Design review of the part built by this model. Coordinates are the model's own, in mm. A direction names the side the tool comes from. Round coordinates to 2 decimals unless told otherwise and drop trailing zeros. Loops run counter-clockwise (first coordinate to the right, second up) from the corner with the lowest first, then second, coordinate; pieces in that order, holes last. Notation, with made-up numbers: (-33.5, -32) - (-27.5, -32) arc R27 ccw to (-27.5, -6) - close; hole circle Ø1 at (32, 69.5). An arc over 180 degrees is marked (long way). Use one line per item in the form item = value. Start each with the question number.
(1) For pin 1 (3 mm diameter, centred on y = -1, z = -6, fed in from -X); pin 2 (2 mm diameter, centred on x = -0.5, z = -5, fed in from -Y); pin 3 (1.9 mm diameter, centred on x = 0, y = 0.5, fed in from +Z); pin 4 (1.1 mm diameter, centred on x = -0.5, z = 2, fed in from -Y), all flat-tipped, find the tip position at first contact; note any pin that passes through.
(2) Wall thickness on probe 1 along Z at (x, y) = (-3, -1); probe 2 along Z at (x, y) = (0.5, -0.75); probe 3 along Y at (x, z) = (-0.75, -18.5): over which ranges is each line inside the solid? List them lowest first. Write a range as [from, to].
(3) We need section B-B, the plane z = -22. Write out the cut boundary in (x, y).
(4) The part is to be moulded in two halves that separate along Y. For faces 1 (the cylindrical face through (-0.455, -3.463, 1.882)), 2 (the flat face through (-1.75, 1.03, 3.68)), 3 (the flat face through (0, 0, 1.27)), 4 (the flat face through (2, 2, 0)), say which applies: released by +Y, released by -Y, zero draft, split by the parting line, or undercut.
(5) Machinability: for faces 5 (the flat face through (1.64, 0.97, 2.4)), 6 (the flat face through (0, 0, -43.561)), 7 (the cylindrical face through (-0.31, 2.33, -21.48)), which of the approach directions +Z, -Z, +X, -X, +Y, -Y give a long, thin tool a straight path to every point of the face, cutting with its end or side? Answer none if there is none.
Autodesk Inventor part; units mm, degrees
ref_plane "YZ Plane" through (0, 0, 0) normal (1, 0, 0) x (0, 1, 0)
ref_plane "XZ Plane" through (0, 0, 0) normal (0, 1, 0) x (-1, 0, 0)
ref_plane "XY Plane" through (0, 0, 0) normal (0, 0, 1) x (1, 0, 0)
sketch "Sketch1" plane through (0, 0, 0) normal (0, 0, 1) x (1, 0, 0)
  circle A0 centre (0, 0) radius 3.4925
  circle A1 centre (0, 0) radius 2.3495
  line L0 (2.1997, 0) -> (1.0999, -1.905)
  line L1 (1.0999, -1.905) -> (-1.0999, -1.905)
  line L2 (-1.0999, -1.905) -> (-2.1997, 0)
  line L3 (-2.1997, 0) -> (-1.0999, 1.905)
  line L4 (-1.0999, 1.905) -> (1.0999, 1.905)
  line L5 (1.0999, 1.905) -> (2.1997, 0)
  dimension "d0" = 6.985
  dimension "d1" = 4.699
  dimension "d2" = 3.81
extrude "Extrusion1" add sketch "Sketch1" along normal blind 3.81 contours A0 | A1
extrude "Extrusion2" add sketch "Sketch1" against normal blind 43.561 contours A1 | L0 L1 L2 L3 L4 L5
extrude "Extrusion3" add sketch "Sketch1" along normal blind 1.27 contours L0 L1 L2 L3 L4 L5
thread "Thread1"
chamfer "Chamfer1" distance 0.254 angle 45 8 edges at (-3.4925, 0, 3.81) (-3.4925, 0, 0) (-1.6498, 0.9525, 3.81) (-1.6498, -0.9525, 3.81) (0, -1.905, 3.81) (1.6498, -0.9525, 3.81) (1.6498, 0.9525, 3.81) (0, 1.905, 3.81)
properties part number "Gearbox Hex Machine Screw" material "Steel"
Data:
q1.pin_1 = -2.35
q1.pin_2 = -2.35
q1.pin_3 = 1.27
q1.pin_4 = -3.49
q2.probe_1 = [0, 3.81]
q2.probe_2 = [-43.56, 1.27]
q2.probe_3 = [-2.23, 2.23]
q3.outline = circle Ø4.7 at (0, 0)
q4.face_1 = split by the parting line
q4.face_2 = undercut
q4.face_3 = undercut
q4.face_4 = zero draft
q5.face_5 = +Z
q5.face_6 = -Z, +X, -X, +Y, -Y
q5.face_7 = -Z
